Source: CAD feature listing. Evaluate the final solid. Frame: model axes, mm. Coordinates: 2 decimals unless noted, no trailing zeros. Write each loop counter-clockwise with the first axis right and the second up, starting at its lowest first coordinate (ties: lowest second). Pieces come first, ordered by that corner, then holes. Notation, with made-up numbers: (26.25, -23.5) - (44.25, -23.5) arc R20 cw to (44.25, -16.5) - close; hole circle Ø6 at (59.25, 59.5). An arc over 180 degrees is marked (long way). One line per item, written item: value.
Autodesk Inventor part; units mm, degrees
ref_plane "YZ Plane" through (0, 0, 0) normal (1, 0, 0) x (0, 1, 0)
ref_plane "XZ Plane" through (0, 0, 0) normal (0, 1, 0) x (-1, 0, 0)
ref_plane "XY Plane" through (0, 0, 0) normal (0, 0, 1) x (1, 0, 0)
sketch "Skizze1" plane through (0, 0, 0) normal (0, 0, 1) x (1, 0, 0)
  line L0 (-37.45, 0) -> (37.45, 0) construction
  line L1 (0, -23.1) -> (0, 23.1) construction
  line L2 (-26.75, -16.5) -> (26.75, -16.5)
  line L3 (26.75, -16.5) -> (26.75, 16.5)
  line L4 (26.75, 16.5) -> (-26.75, 16.5)
  line L5 (-26.75, 16.5) -> (-26.75, -16.5)
  line L6 (-26.75, -16.5) -> (26.75, 16.5) construction
  line L7 (26.75, -16.5) -> (-26.75, 16.5) construction
  circle A0 centre (-23.25, -8.25) radius 1.5
  circle A1 centre (23.25, -8.25) radius 1.5
  circle A2 centre (-23.25, 8.25) radius 1.5
  circle A3 centre (23.25, 8.25) radius 1.5
  point P0 (0, 0)
  dimension "d0" = 53.5
  dimension "d1" = 33
  dimension "d4" = 3
  dimension "d7" = 8.25
  dimension "d8" = 23.25
extrude "Extrusion1" add sketch "Skizze1" along normal blind 3.5
properties part number "LC_mirror_holder_back"
1) Section query A-A on z = 2.6. Output: boundary loops of the cut face in (x, y).
Values found:
outline: (-26.75, -16.5) - (26.75, -16.5) - (26.75, 16.5) - (-26.75, 16.5) - close; hole circle Ø3 at (-23.25, -8.25); hole circle Ø3 at (-23.25, 8.25); hole circle Ø3 at (23.25, -8.25); hole circle Ø3 at (23.25, 8.25)
2) Draft query along X for faces 1 (the flat face through (-26.75, 0, 2)), 2 (the flat face through (26.75, 0, 2)), 3 (the flat face through (0, 0, 3.5)), 4 (the cylindrical face through (22.06, 9.16, 1.73)). Return one class per face: released by +X, released by -X, zero draft, split by the parting line, or undercut.
Values found:
face 1: released by -X
face 2: released by +X
face 3: zero draft
face 4: undercut
3) Section query B-B on x = 23.25. Output: boundary loops of the cut face in (y, z).
Values found:
outline: (-16.5, 0) - (-9.75, 0) - (-9.75, 3.5) - (-16.5, 3.5) - close; (-6.75, 0) - (6.75, 0) - (6.75, 3.5) - (-6.75, 3.5) - close; (9.75, 0) - (16.5, 0) - (16.5, 3.5) - (9.75, 3.5) - close
4) Section query C-C on y = 8.25. Output: boundary loops of the cut face in (x, z), then the cut area to 3 significant figures.
Values found:
outline: (-26.75, 0) - (-24.75, 0) - (-24.75, 3.5) - (-26.75, 3.5) - close; (-21.75, 0) - (21.75, 0) - (21.75, 3.5) - (-21.75, 3.5) - close; (24.75, 0) - (26.75, 0) - (26.75, 3.5) - (24.75, 3.5) - close
area: 166 mm2
5) Material intervals for line 1 (Y direction, x = -23.25, z = 1.4); line 2 (X direction, y = 7.5, z = 0.45); line 3 (X direction, y = 9.5, z = 1.65), sorted ascending.
Values found:
line 1: -16.5 to -9.75, -6.75 to 6.75, 9.75 to 16.5
line 2: -26.75 to -24.55, -21.95 to 21.95, 24.55 to 26.75
line 3: -26.75 to -24.08, -22.42 to 22.42, 24.08 to 26.75
